from build123d import *

# Parameters (mm, degrees)
F0_R      = 12.5
F1_DEPTH  = 1.5
F2_R      = 7.5
F3_DEPTH  = 1
F4_R      = 7.75
F5_DEPTH  = 1
F6_R      = 7.5
F7_DEPTH  = 2
F9_R      = 1.75
F10_DEPTH = 5.501
F11_R     = 0.125


with BuildPart() as f1:
    # F0 (on Top) → F1 (new body)
    with BuildSketch(Plane.XY):
        Circle(F0_R)
    extrude(amount=F1_DEPTH)

    # F2 (on face) → F3 (join)
    with BuildSketch(Plane.XY.offset(1.5)):
        Circle(F2_R)
    extrude(amount=F3_DEPTH)

    # F4 (on face) → F5 (join)
    with BuildSketch(Plane.XY.offset(2.5)):
        Circle(F4_R)
    extrude(amount=F5_DEPTH)

    # F6 (on face) → F7 (join)
    with BuildSketch(Plane.XY.offset(3.5)):
        Circle(F6_R)
    extrude(amount=F7_DEPTH)

    # F9 (on face) → F10 (cut, through all)
    with BuildSketch(Plane.XY.offset(5.5)):
        Circle(F9_R)
    extrude(amount=-F10_DEPTH, mode=Mode.SUBTRACT)

    # F11
    f11_edges = [f1.edges().sort_by_distance(p)[0] for p in [
        (-7.75, 0, 3.5),
        (-7.75, 0, 2.5),
    ]]
    fillet(f11_edges, radius=F11_R)


solid = f1.part
Geometry check sheet. Reference: the model listing, model coordinates, mm. A direction names the side the tool comes from. Give positions to 0.01 mm unless a question says otherwise; leave off trailing zeros. Order: outer loops, then holes, each group sorted by start corner. A loop starts at its lowest first (then second) coordinate and runs counter-clockwise, first axis right, second up. Notation, with made-up numbers: M 34,-4.75 L 90,-4.75 A24 ccw 90,19.25 Z; hole C -29,44.25 d3. An arc over 180 degrees is marked long. Use a Markdown table: item, result.
Item 1: Section check A-A (y = 0). Record the cut outline in (x, z) (3 decimals), and give its area (3 significant figures).
Answers follow:
| item | result |
|---|---|
| outline | M -12.5,0 L -1.75,0 L -1.75,5.5 L -7.5,5.5 L -7.5,3.5 L -7.625,3.5 A0.125 ccw -7.75,3.375 L -7.75,2.625 A0.125 ccw -7.625,2.5 L -7.5,2.5 L -7.5,1.5 L -12.5,1.5 Z; M 1.75,0 L 12.5,0 L 12.5,1.5 L 7.5,1.5 L 7.5,2.5 L 7.625,2.5 A0.125 ccw 7.75,2.625 L 7.75,3.375 A0.125 ccw 7.625,3.5 L 7.5,3.5 L 7.5,5.5 L 1.75,5.5 Z |
| area | 78.7 mm2 |
Item 2: Section check C-C (z = 0.4). Record the cut outline in (x, y), and give its area (3 significant figures).
Answers follow:
| item | result |
|---|---|
| outline | C 0,0 d25; hole C 0,0 d3.5 |
| area | 481 mm2 |
Item 3: Draft check along X on faces 4 (the flat face through (0, 2, 5.5)), 5 (the cylindrical face through (-1.009, 7.684, 2.995)), 6 (the cylindrical face through (1.617, -0.67, 2.788)). Enter one of: +X half, -X half, draft (parallel to the pull), parting line (faces both ways), or undercut.
Answers follow:
| item | result |
|---|---|
| face 4 | draft |
| face 5 | parting line |
| face 6 | undercut |
Item 4: Depth check by flat-ended pin: P1, Ø3, axis at y = 8, z = 1.5, coming from the +X side. Enter the tip coordinate at first touch or a pass-through.
Answers follow:
| item | result |
|---|---|
| P1 | stops at x = 10.68 |
Item 5: Material ranges on line 1 along Y through (x, z) = (0, 3.7); line 2 along Y through (x, z) = (0, 2.6); line 3 along Z through (x, y) = (7, 8.75), recorded low to high.
Answers follow:
| item | result |
|---|---|
| line 1 | y = -7.5 to -1.75, 1.75 to 7.5 |
| line 2 | y = -7.75 to -1.75, 1.75 to 7.75 |
| line 3 | z = 0 to 1.5 |
Item 6: Section check D-D (x = 9.5). Record the cut outline in (y, z), and give its area (3 significant figures).
Answers follow:
| item | result |
|---|---|
| outline | M -8.12,0 L 8.12,0 L 8.12,1.5 L -8.12,1.5 Z |
| area | 24.4 mm2 |
Item 7: Tool access check on faces 1 (the cylindrical face through (-7.493, 0.33, 1.993)), 2 (the flat face through (0, -3, 0)), 3 (the cylindrical face through (-7.493, 0.33, 4.486)). Record the directions out of +Z, -Z, +X, -X, +Y, -Y that give a thin tool (end or side, any length) a straight path to the whole face; none if there is none.
Answers follow:
| item | result |
|---|---|
| face 1 | none |
| face 2 | -Z, +X, -X, +Y, -Y |
| face 3 | +Z |
